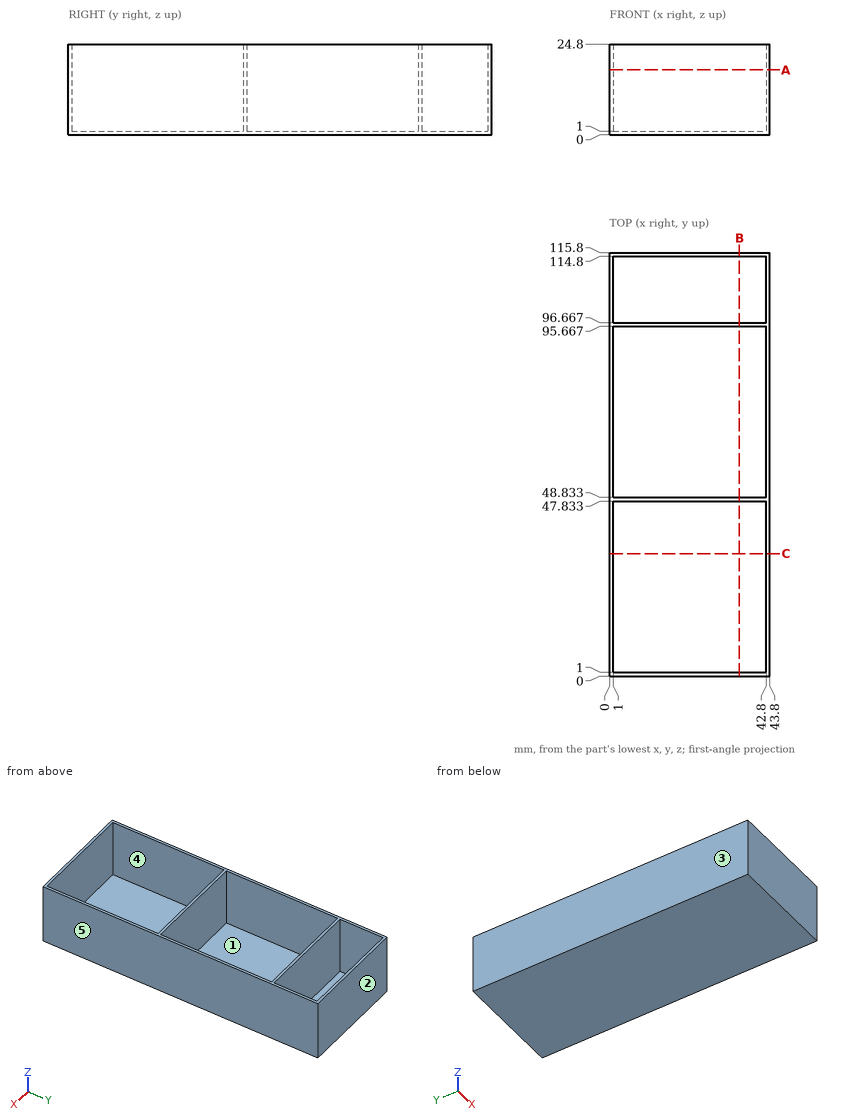
The drawing under review shows one solid part. Ordinate dimensions are in mm from its lowest x, y, z. A direction names the side the tool comes from. Coordinates: 2 decimals unless noted, no trailing zeros. Write each loop counter-clockwise with the first axis right and the second up, starting at its lowest first coordinate (ties: lowest second). Pieces come first, ordered by that corner, then holes. Notation, with made-up numbers: (77.5, 49.5) -> (81.5, 49.5) arc R31 ccw to (81.5, 86.5) -> close; hole circle Ø10 at (1.25, 74.5). An arc over 180 degrees is marked (long way). One line per item, written item: value. Start each with the question number.
Q1. To check wall thickness, follow probe 1 along Y at (x, z) = (29.5, 15.5); probe 2 along X at (y, z) = (87, 22.5); probe 3 along Z at (x, y) = (24, 38.5). State the ranges of each line that lie inside material, in increasing order.
Q2. For the marked faces 4 and 5, list the 3-axis set-ups (+Z, -Z, +X, -X, +Y, -Y) from which the entire face can be reached by the end or side of a thin tool; tool diameter is ignored.
Q3. Add section C-C, the plane y = 33.5. Give the boundary of the cut face in (x, z).
Q4. Add section B-B, the plane x = 35.5. Give the boundary of the cut face in (y, z).
Q5. Clearance check with flat-ended pins moving along their axes: P1, Ø12, axis at x = 20.5, z = 16.5, coming from the -Y side; P2, Ø5, axis at x = 20.5, y = 101.5, coming from the +Z side. State where each tip first meets the part, or that it passes through.
Q6. The part is to be moulded in two halves that separate along X. For the marked faces 1, 2 and 3, say which applies: +X half, -X half, draft (parallel to the pull), parting line (faces both ways), or undercut.
Q7. Add section A-A, the plane z = 17.75. Give the boundary of the cut face in (x, y).
Response:
1. probe 1: 0 to 1, 47.83 to 48.83, 95.67 to 96.67, 114.8 to 115.8
1. probe 2: 0 to 1, 42.8 to 43.8
1. probe 3: 0 to 1
2. face 4: +Z
2. face 5: +Z, -Z, +X, +Y, -Y
3. outline: (0, 0) -> (43.8, 0) -> (43.8, 24.8) -> (42.8, 24.8) -> (42.8, 1) -> (1, 1) -> (1, 24.8) -> (0, 24.8) -> close
4. outline: (0, 0) -> (115.8, 0) -> (115.8, 24.8) -> (114.8, 24.8) -> (114.8, 1) -> (96.67, 1) -> (96.67, 24.8) -> (95.67, 24.8) -> (95.67, 1) -> (48.83, 1) -> (48.83, 24.8) -> (47.83, 24.8) -> (47.83, 1) -> (1, 1) -> (1, 24.8) -> (0, 24.8) -> close
5. P1: y = 0
5. P2: z = 1
6. face 1: undercut
6. face 2: draft
6. face 3: -X half
7. outline: (0, 0) -> (43.8, 0) -> (43.8, 115.8) -> (0, 115.8) -> close; hole (1, 1) -> (42.8, 1) -> (42.8, 47.83) -> (1, 47.83) -> close; hole (1, 48.83) -> (42.8, 48.83) -> (42.8, 95.67) -> (1, 95.67) -> close; hole (1, 96.67) -> (42.8, 96.67) -> (42.8, 114.8) -> (1, 114.8) -> close
